from build123d import *

# Parameters (mm, degrees)
SKETCH1_R           = 11.43
BOSS_EXTRUDE1_DEPTH = 6.35
SKETCH2_R           = 3.4925
CUT_EXTRUDE1_DEPTH  = 69.453471241
SKETCH3_R           = 1
CUT_EXTRUDE2_DEPTH  = 80.463850272


with BuildPart() as part:
    # Sketch1 → Boss-Extrude1 (new, symmetric)
    with BuildSketch(Plane.XY):
        Polygon((-38.1, 0), (38.1, 0), (38.1, 3.175), (5.588, 3.175), (5.588, 31.75), (13.97, 31.75), (13.97, 59.69), (-13.97, 59.69), (-13.97, 31.75), (-5.588, 31.75), (-5.588, 3.175), (-38.1, 3.175), align=None)
        with Locations((0, 45.72)):
            Circle(SKETCH1_R, mode=Mode.SUBTRACT)
    extrude(amount=BOSS_EXTRUDE1_DEPTH, both=True)

    # Sketch2 → Cut-Extrude1 (cut, through all)
    with BuildSketch(Plane(origin=(0, 3.175, 0), x_dir=(1, 0, 0), z_dir=(0, 1, 0))):
        with Locations(Location((-31.75, 0, 0), (0, 0, 180))):
            Circle(SKETCH2_R)
        with Locations(Location((31.75, 0, 0), (0, 0, 180))):
            Circle(SKETCH2_R)
        with Locations(Location((-12.7, 0, 0), (0, 0, 180))):
            Circle(SKETCH2_R)
        with Locations(Location((12.7, 0, 0), (0, 0, 180))):
            Circle(SKETCH2_R)
    extrude(amount=-CUT_EXTRUDE1_DEPTH, mode=Mode.SUBTRACT)

    # Sketch3 → Cut-Extrude2 (cut, through all)
    with BuildSketch(Plane(origin=(13.97, 0, 0), x_dir=(0, 0, -1), z_dir=(1, 0, 0))):
        with Locations((0, 45.72)):
            Circle(SKETCH3_R)
    extrude(amount=-CUT_EXTRUDE2_DEPTH, mode=Mode.SUBTRACT)


solid = part.part
Could you check a few things on this model? Use its own coordinates, in mm. A direction names the side the tool comes from. Give positions to 0.01 mm unless a question says otherwise; leave off trailing zeros. Order: outer loops, then holes, each group sorted by start corner. A loop starts at its lowest first (then second) coordinate and runs counter-clockwise, first axis right, second up.
1. We'd pull the mould along Y, two halves only. Please class faces 5 (the cylindrical face through (-12.66, 44.744, 0.217)), 6 (the flat face through (-1, 0, 0)), 7 (the flat face through (-38.1, 2, 0)): pulls with the +Y half, pulls with the -Y half, needs draft (parallel to the pull), parting line crosses it, or undercut.
2. I need wall thicknesses on L1, parallel to Z at x = -31.75, y = 2.4; L2, parallel to Y at x = -12.8, z = 0; L3, parallel to X at y = 32.5, z = -5.5. Which ranges of each line are inside material? Lowest first, please.
3. For faces 1 (the flat face through (-13.97, 46, 2)), 2 (the flat face through (-5.588, 18, 0)), 3 (the cylindrical face through (-9.21, 1.61, 0.15)), 4 (the flat face through (5.588, 17, 0)), which set-ups out of +Z, -Z, +X, -X, +Y, -Y let a thin tool reach every point of the face, with its end or its side?
4. Suppose I cut it at D-D (z = -5.5). List the corners of the cut face in (x, y) for me (3 decimals), plus the area to 4 significant figures.
5. Will these pins go through, and if not, where does the flat tip stop? P1, Ø4, axis at y = 24.5, z = 3, coming from the -X side; P2, Ø4, axis at x = -26, z = 0, coming from the +Y side (3 decimals); P3, Ø4, axis at y = 50, z = 1.5, coming from the +X side; P4, Ø12, axis at x = -10, y = 30.5, coming from the +Z side.
6. Suppose I cut it at B-B (x = -12.7). Give the number of separate pieces and of enclosed holes in the cut face, plus the area to 3 significant figures.
7. Suppose I cut it at A-A (y = 45.72). List the corners of the cut face in (x, z) for me.
Solved:
1. face 5: undercut
1. face 6: pulls with the -Y half
1. face 7: needs draft
2. L1: z = -6.35 to -3.49, 3.49 to 6.35
2. L2: y = 31.75 to 44.72, 46.72 to 59.69
2. L3: x = -13.97 to 13.97
3. face 1: +Z, -Z, -X, +Y
3. face 2: +Z, -Z, -X
3. face 3: -Y
3. face 4: +Z, -Z, +X
4. outline: (-38.1, 0) - (38.1, 0) - (38.1, 3.175) - (5.588, 3.175) - (5.588, 31.75) - (13.97, 31.75) - (13.97, 59.69) - (-13.97, 59.69) - (-13.97, 31.75) - (-5.588, 31.75) - (-5.588, 3.175) - (-38.1, 3.175) - close; hole circle Ø22.86 at (0, 45.72)
4. area: 931.5 mm2
5. P1: stops at x = -5.59
5. P2: stops at y = 3.175
5. P3: stops at x = 13.97
5. P4: stops at z = 6.35
6. separate pieces: 3
6. enclosed holes: 1
6. area: 370 mm2
7. outline: (-13.97, -6.35) - (-11.43, -6.35) - (-11.43, -1) - (-13.97, -1) - close; (-13.97, 1) - (-11.43, 1) - (-11.43, 6.35) - (-13.97, 6.35) - close; (11.43, -6.35) - (13.97, -6.35) - (13.97, -1) - (11.43, -1) - close; (11.43, 1) - (13.97, 1) - (13.97, 6.35) - (11.43, 6.35) - close
